The model under review builds one solid part; all positions refer to its coordinate system, in mm. Face numbers are marked on the shaded views. A direction names the side the tool comes from. Give positions to 0.01 mm unless a question says otherwise; leave off trailing zeros. Order: outer loops, then holes, each group sorted by start corner. A loop starts at its lowest first (then second) coordinate and runs counter-clockwise, first axis right, second up. Notation, with made-up numbers: (68.25, 30.25) -> (80.25, 30.25) arc R10 ccw to (80.25, 49.25) -> close; hole circle Ø4 at (23, 34). An arc over 180 degrees is marked (long way). Use one line per item in the form item = value.
```python
from build123d import *

# Parameters (mm, degrees)
SKETCH_1_R      = 12.5
SKETCH_1_R_2    = 2
EXTRUDE_1_DEPTH = 4
SKETCH_2_R      = 12.5
SKETCH_2_R_2    = 3.75
EXTRUDE_2_DEPTH = 3


with BuildPart() as part:
    # 草图1 → 凸台-拉伸1 (new body)
    with BuildSketch(Plane.XY):
        Circle(SKETCH_1_R)
        with Locations((0, 8)):
            Circle(SKETCH_1_R_2, mode=Mode.SUBTRACT)
        with Locations((6.92820323, -4)):
            Circle(SKETCH_1_R_2, mode=Mode.SUBTRACT)
        with Locations((-6.92820323, -4)):
            Circle(SKETCH_1_R_2, mode=Mode.SUBTRACT)
    extrude(amount=EXTRUDE_1_DEPTH)

    # 草图2 → 凸台-拉伸2 (add)
    with BuildSketch(Plane.XY.offset(4)):
        Circle(SKETCH_2_R)
        with Locations((0, 8)):
            Circle(SKETCH_2_R_2, mode=Mode.SUBTRACT)
        with Locations((6.92820323, -4)):
            Circle(SKETCH_2_R_2, mode=Mode.SUBTRACT)
        with Locations((-6.92820323, -4)):
            Circle(SKETCH_2_R_2, mode=Mode.SUBTRACT)
    extrude(amount=EXTRUDE_2_DEPTH)


solid = part.part
```
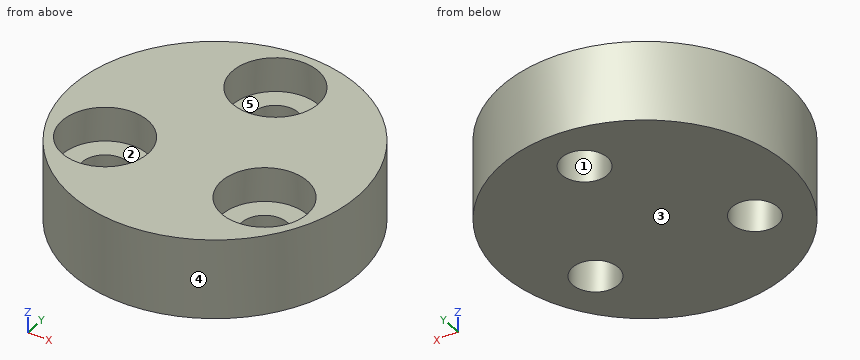
1. Tool access review of the marked faces 1 and 2: name each direction out of +Z, -Z, +X, -X, +Y, -Y from which nothing blocks a thin tool from reaching the whole face with its end or side.
Values:
face_1 = +Z, -Z
face_2 = +Z
2. For L1, parallel to Y at x = 0, z = 1.8; L2, parallel to X at y = -2.75, z = 6.25; L3, parallel to Z at x = -4.5, y = -2.5, list the stretches that pass through material, from the lowest coordinate up.
Values:
L1 = -12.5 to 6, 10 to 12.5
L2 = -12.19 to -10.46, -3.39 to 3.39, 10.46 to 12.19
L3 = 0 to 4
3. Add section C-C on y = -4. Give the boundary of the cut face in (x, z), then the cut area to 3 significant figures.
Values:
outline = (-11.84, 0) -> (-8.93, 0) -> (-8.93, 4) -> (-10.68, 4) -> (-10.68, 7) -> (-11.84, 7) -> close; (-4.93, 0) -> (4.93, 0) -> (4.93, 4) -> (3.18, 4) -> (3.18, 7) -> (-3.18, 7) -> (-3.18, 4) -> (-4.93, 4) -> close; (8.93, 0) -> (11.84, 0) -> (11.84, 7) -> (10.68, 7) -> (10.68, 4) -> (8.93, 4) -> close
area = 88.8 mm^2
4. Add section D-D on z = 5.5. Give the boundary of the cut face in (x, y), then the cut area to 3 significant figures.
Values:
outline = circle Ø25 at (0, 0); hole circle Ø7.5 at (-6.93, -4); hole circle Ø7.5 at (0, 8); hole circle Ø7.5 at (6.93, -4)
area = 358 mm^2
5. Add section A-A on x = 0. Give the boundary of the cut face in (y, z).
Values:
outline = (-12.5, 0) -> (6, 0) -> (6, 4) -> (4.25, 4) -> (4.25, 7) -> (-12.5, 7) -> close; (10, 0) -> (12.5, 0) -> (12.5, 7) -> (11.75, 7) -> (11.75, 4) -> (10, 4) -> close
6. The part is to be moulded in two halves that separate along Y. For the marked faces 3, 4 and 5, say which applies: +Y half, -Y half, draft (parallel to the pull), parting line (faces both ways), or undercut.
Values:
face_3 = draft
face_4 = parting line
face_5 = undercut
7. Add section B-B on y = 8. Give the boundary of the cut face in (x, z), then the cut area to 3 significant figures.
Values:
outline = (-9.6, 0) -> (-2, 0) -> (-2, 4) -> (-3.75, 4) -> (-3.75, 7) -> (-9.6, 7) -> close; (2, 0) -> (9.6, 0) -> (9.6, 7) -> (3.75, 7) -> (3.75, 4) -> (2, 4) -> close
area = 96.0 mm^2
8. For pin 1 Ø3 at (x, z) = (-4, 6) entering from -Y; pin 2 Ø4.5 at (x, y) = (6.93, -4) entering from +Z; pin 3 Ø4 at (y, z) = (8, 5.5) entering from -X, all flat-tipped, find the tip position at first contact; note any pin that passes through.
Values:
pin_1 = -12.25
pin_2 = 4
pin_3 = -10.97
